Geometry check sheet. Reference: the model listing, model coordinates, mm. A direction names the side the tool comes from. Coordinates: 2 decimals unless noted, no trailing zeros. Order: outer loops, then holes, each group sorted by start corner. A loop starts at its lowest first (then second) coordinate and runs counter-clockwise, first axis right, second up. Notation, with made-up numbers: (-19, -6.75) - (-6, -6.75) arc R28 cw to (-6, 12.25) - close; hole circle Ø3 at (6, -28). An arc over 180 degrees is marked (long way). Return JSON: item names as keys, results as strings. Group by question number.
Item 1: Section check C-C on x = 0. Enter the section's corners in (y, z) (3 decimals), then the cut area to 3 significant figures.
Item 2: Draft check along Z on faces 1 (the flat face through (0, 47, 19)), 2 (the flat face through (14.21, 45.52, 15.51)), 3 (the cylindrical face through (-0.29, 45.52, 27.75)), 4 (the conical face through (-0.209, 46.815, -12.838)). Enter one of: pulls with the +Z half, pulls with the -Z half, needs draft (parallel to the pull), parting line crosses it, or undercut.
Item 3: Scan lines: probe 1 along Z at (x, y) = (0, 36.25) (3 decimals); probe 2 along Y at (x, z) = (11.5, 14); probe 3 along Z at (x, y) = (9, 37.25). Record each from-to range of solid material in increasing order.
Item 4: Section check D-D on y = 32. Enter the section's corners in (x, z) (3 decimals).
Item 5: Tool access check on faces 5 (the conical face through (0.209, 46.815, 12.838)), 6 (the flat face through (-14.21, 45.52, 15.51)), 7 (the flat face through (-13, 45, -5.15)). Record the directions out of +Z, -Z, +X, -X, +Y, -Y that give a thin tool (end or side, any length) a straight path to the whole face; none if there is none.
Item 6: Section check B-B on z = 0. Enter the section's corners in (x, y) (3 decimals), then the cut area to 3 significant figures.
Item 7: Gauge pin test, flat ends, axial feed: pin 1 (1 mm diameter, centred on x = 12.5, y = 45, fed in from +Z); pin 2 (1.5 mm diameter, centred on x = -12, y = 45, fed in from +Z); pin 3 (3 mm diameter, centred on x = -12.5, z = -1, fed in from +Y); pin 4 (2 mm diameter, centred on x = -8.5, z = 7.5, fed in from -Y). Record the tip position at first contact, or that the pin passes through.
Item 8: Section check A-A on y = 44.75. Enter the section's corners in (x, z) (3 decimals), then the cut area to 3 significant figures.
from build123d import *

# Parameters (mm, degrees)
SKETCH136_R             = 14.5
PAD078_DEPTH            = 17.5
PAD079_DEPTH            = 1.5
SKETCH138_R             = 12.725
POCKET051_DEPTH         = 18.501
CHAMFER_SIZE            = 0.3
CHAMFER001_SIZE         = 0.3
SKETCH_W                = 30
SKETCH_H                = 10.3
POCKET_DEPTH            = 3.75
BODY028_PLACEMENT_ANGLE = 90


with BuildPart() as part:
    # Sketch136 → Pad078 (new body)
    with BuildSketch(Plane.XY.offset(18.5)):
        Circle(SKETCH136_R)
    extrude(amount=-PAD078_DEPTH)

    # Sketch141 → Pad079 (join, symmetric)
    with BuildSketch(Plane.XY.offset(17)):
        with BuildLine():
            Line((0, 0), (18.747628, -20.459446))
            ThreePointArc((-18.747628, -20.459446), (0, -27.75), (18.747628, -20.459446))
            Line((0, 0), (-18.747628, -20.459446))
        make_face()
    extrude(amount=PAD079_DEPTH, both=True)

    # Sketch138 → Pocket051 (cut, through all)
    with BuildSketch(Plane.XY):
        Circle(SKETCH138_R)
    extrude(amount=POCKET051_DEPTH, mode=Mode.SUBTRACT)

    # Chamfer
    chamfer_edges = [part.edges().sort_by_distance(p)[0] for p in [
        (-12.725, 0, 1),
        (-14.5, 0, 1),
    ]]
    chamfer(chamfer_edges, length=CHAMFER_SIZE)

    # Chamfer001
    chamfer001_edges = [part.edges().sort_by_distance(p)[0] for p in [
        (0, -12.725, 18.5),
    ]]
    chamfer(chamfer001_edges, length=CHAMFER001_SIZE)

    # Sketch → Pocket (cut)
    with BuildSketch(Plane.XY.offset(18.5)):
        Rectangle(SKETCH_W, SKETCH_H)
    extrude(amount=-POCKET_DEPTH, mode=Mode.SUBTRACT)


with BuildPart() as part_1:
    # Body028 placement: moved
    add(part.part.moved(Location((0, 28.5, 0))).rotate(Axis((0, 28.5, 0), (-1, 0, 0)), BODY028_PLACEMENT_ANGLE))


solid = part_1.part
Computed:
{
 "1": {"outline": "(29.5, -14.2) - (29.8, -14.5) - (47, -14.5) - (47, -13.025) - (46.7, -12.725) - (29.8, -12.725) - (29.5, -13.025) - close; (29.5, 13.025) - (29.8, 12.725) - (46.7, 12.725) - (47, 13.025) - (47, 27.75) - (44, 27.75) - (44, 14.5) - (29.8, 14.5) - (29.5, 14.2) - close", "area": "102 mm²"},
 "2": {"face 1": "needs draft", "face 2": "undercut", "face 3": "pulls with the +Z half", "face 4": "undercut"},
 "3": {"probe 1": "z = -14.5 to -12.725, 12.725 to 14.5", "probe 2": "y = 44 to 47", "probe 3": "z = -11.37 to -9, 9 to 11.37"},
 "4": {"outline": "circle Ø29 at (0, 0); hole circle Ø25.45 at (0, 0)"},
 "5": {"face 5": "+Y", "face 6": "-X, +Y, -Y", "face 7": "+X, -X, +Y"},
 "6": {"outline": "(-14.5, 29.8) - (-14.2, 29.5) - (-13.025, 29.5) - (-12.725, 29.8) - (-12.725, 43.25) - (-14.5, 43.25) - close; (12.725, 29.8) - (13.025, 29.5) - (14.2, 29.5) - (14.5, 29.8) - (14.5, 43.25) - (12.725, 43.25) - close", "area": "48.6 mm²"},
 "7": {"pin 1": "stops at z = 25.02", "pin 2": "stops at z = 25.37", "pin 3": "stops at y = 43.25", "pin 4": "passes through"},
 "8": {"outline": "(-18.748, 20.459) - (-9.796, 10.691) arc R14.5 ccw to (-13.555, 5.15) - (-11.636, 5.15) arc R12.725 cw to (11.636, 5.15) - (13.555, 5.15) arc R14.5 ccw to (9.796, 10.691) - (18.748, 20.459) arc R27.75 ccw to start; (-13.555, -5.15) arc R14.5 ccw to (13.555, -5.15) - (11.636, -5.15) arc R12.725 cw to (-11.636, -5.15) - close", "area": "530 mm²"}
}
